Could you check a few things on this drawing? It's one solid part, dimensions in mm from its lowest x, y, z. A direction names the side the tool comes from. Coordinates: 2 decimals unless noted, no trailing zeros. Write each loop counter-clockwise with the first axis right and the second up, starting at its lowest first coordinate (ties: lowest second). Pieces come first, ordered by that corner, then holes.
Item 1: I want a section at A-A (z = 65). Please give me the cut outline in (x, y).
Item 2: For the marked faces 4 and 5, which set-ups out of +Z, -Z, +X, -X, +Y, -Y let a thin tool reach every point of the face, with its end or its side?
Item 3: I want a section at B-B (x = 614). Please give me the cut outline in (y, z), and give its area (3 significant figures).
Item 4: I'm going to push flat-ended pins straight in: P1, Ø10, axis at y = 80.5, z = 75.5, coming from the -X side; P2, Ø1.5, axis at x = 712.5, y = 71.5, coming from the -Z side; P3, Ø16, axis at x = 575.5, y = 76, coming from the -Z side. Where does each tip first touch, or does it pass through?
Item 5: I want a section at C-C (z = 111). Please give me the cut outline in (x, y).
Item 6: If we mould it in two halves opening along Y, with no side actions, what happens to the marked faces 1, 2 and 3? For each: pulls with the +Y half, pulls with the -Y half, needs draft (parallel to the pull), parting line crosses it, or undercut.
Item 7: Please list where these lines run through material, in increasing order: line 1 (Z direction, x = 175, y = 76); line 2 (Y direction, x = 691, z = 129.5); line 3 (X direction, y = 74, z = 46).
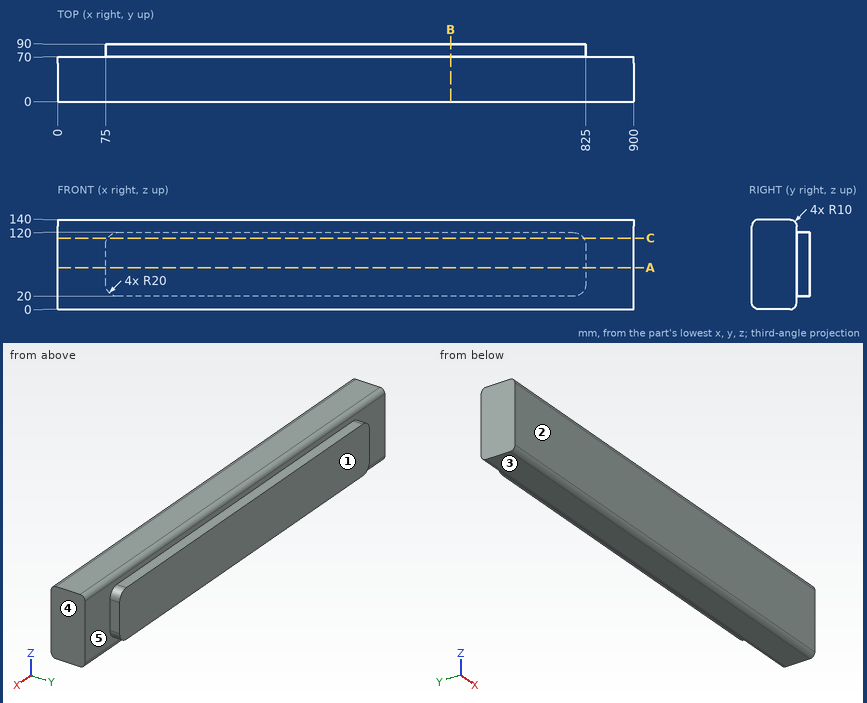
Answer:
1. outline: (0, 0) - (900, 0) - (900, 70) - (825, 70) - (825, 90) - (75, 90) - (75, 70) - (0, 70) - close
2. face 4: +Z, -Z, +X, +Y, -Y
2. face 5: +Y
3. outline: (0, 10) arc R10 ccw to (10, 0) - (60, 0) arc R10 ccw to (70, 10) - (70, 20) - (90, 20) - (90, 120) - (70, 120) - (70, 130) arc R10 ccw to (60, 140) - (10, 140) arc R10 ccw to (0, 130) - close
3. area: 11,700 mm2
4. P1: stops at x = 75
4. P2: stops at z = 20
4. P3: stops at z = 4
5. outline: (0, 0) - (900, 0) - (900, 70) - (821.7, 70) - (821.7, 90) - (78.3, 90) - (78.3, 70) - (0, 70) - close
6. face 1: pulls with the +Y half
6. face 2: pulls with the -Y half
6. face 3: needs draft
7. line 1: z = 20 to 120
7. line 2: y = 0 to 70
7. line 3: x = 75 to 825
